```python
from build123d import *

# Parameters (mm, degrees)
SKETCH1_W           = 66.04
SKETCH1_H           = 147.574
BOSS_EXTRUDE1_DEPTH = 3.03784
SKETCH3_W           = 66.04
SKETCH3_H           = 3.03784
BOSS_EXTRUDE2_DEPTH = 16.51
SKETCH4_R           = 3.3782
CUT_EXTRUDE1_DEPTH  = 163.854183627
SKETCH5_R           = 2.5527
CUT_EXTRUDE2_DEPTH  = 3.03784
BASE_FLANGE1_START  = -66.04
BASE_FLANGE1_DEPTH  = 66.04
SKETCH11_R          = 3.3782
CUT_EXTRUDE3_DEPTH  = 163.854183627
SKETCH12_R          = 2.2479
CUT_EXTRUDE4_DEPTH  = 163.517528827
CUT_EXTRUDE6_DEPTH  = 1.51892
EDGE_FLANGE1_DEPTH  = 128.79832


# Read off the part's stored shape, not the designer's step: Base-Flange1
# Sheet-metal steps are written as plain solids
with BuildPart() as part:
    # Sketch1 → Boss-Extrude1 (new body)
    with BuildSketch(Plane.XY):
        with Locations((33.02, 73.787)):
            Rectangle(SKETCH1_W, SKETCH1_H)
    extrude(amount=BOSS_EXTRUDE1_DEPTH)

    # Sketch3 → Boss-Extrude2 (add)
    with BuildSketch(Plane.XY.offset(3.03784)):
        with Locations((33.02, 146.05508)):
            Rectangle(SKETCH3_W, SKETCH3_H)
        with Locations((33.02, 1.51892)):
            Rectangle(SKETCH3_W, SKETCH3_H)
    extrude(amount=BOSS_EXTRUDE2_DEPTH)

    # Sketch4 → Cut-Extrude1 (cut, through all)
    with BuildSketch(Plane.XZ):
        with Locations(Location((12.7, 12.68984, 0), (0, 0, 270))):
            Circle(SKETCH4_R)
        with Locations(Location((53.34, 12.68984, 0), (0, 0, 270))):
            Circle(SKETCH4_R)
    extrude(amount=-CUT_EXTRUDE1_DEPTH, mode=Mode.SUBTRACT)

    # Sketch5 → Cut-Extrude2 (cut)
    with BuildSketch(Plane.XY.offset(3.03784)):
        with Locations((46.99, 126.449057869)):
            Circle(SKETCH5_R)
        with Locations((19.05, 126.449057869)):
            Circle(SKETCH5_R)
        with Locations((6.35, 75.141057869)):
            Circle(SKETCH5_R)
        with Locations((59.69, 75.141057869)):
            Circle(SKETCH5_R)
    extrude(amount=-CUT_EXTRUDE2_DEPTH, mode=Mode.SUBTRACT)


with BuildPart() as body_2:
    # Base-Flange1 outline → Base-Flange1 (new body)
    with BuildSketch(Plane.ZY.offset(BASE_FLANGE1_START)):
        with BuildLine():
            ThreePointArc((1.51892, 4.94284), (2.52176295, 2.52176295), (4.94284, 1.51892))
            Line((4.94284, 1.51892), (19.54784, 1.51892))
            Line((19.54784, 1.51892), (19.54784, 3.03784))
            Line((19.54784, 3.03784), (4.94284, 3.03784))
            ThreePointArc((4.94284, 3.03784), (3.595801582, 3.595801582), (3.03784, 4.94284))
            Line((3.03784, 4.94284), (3.03784, 142.63116))
            ThreePointArc((3.03784, 142.63116), (3.595801582, 143.978198418), (4.94284, 144.53616))
            Line((4.94284, 144.53616), (19.54784, 144.53616))
            Line((19.54784, 144.53616), (19.54784, 146.05508))
            Line((19.54784, 146.05508), (4.94284, 146.05508))
            ThreePointArc((4.94284, 146.05508), (2.52176295, 145.05223705), (1.51892, 142.63116))
            Line((1.51892, 142.63116), (1.51892, 4.94284))
        make_face()
    extrude(amount=BASE_FLANGE1_DEPTH)

    # Sketch11 → Cut-Extrude3 (cut, through all)
    with BuildSketch(Plane.XZ):
        with Locations((53.34, 12.68984)):
            Circle(SKETCH11_R)
        with Locations((12.7, 12.68984)):
            Circle(SKETCH11_R)
    extrude(amount=-CUT_EXTRUDE3_DEPTH, mode=Mode.SUBTRACT)

    # Sketch12 → Cut-Extrude4 (cut, through all)
    with BuildSketch(Plane.XY.offset(3.03784)):
        with Locations((55.9637, 77.009977807)):
            Circle(SKETCH12_R)
        with Locations((9.8441, 77.009977807)):
            Circle(SKETCH12_R)
        with Locations((46.993900058, 128.317977807)):
            Circle(SKETCH12_R)
        with Locations((19.053900058, 128.317977807)):
            Circle(SKETCH12_R)
    extrude(amount=-CUT_EXTRUDE4_DEPTH, mode=Mode.SUBTRACT)

    # Sketch14 → Cut-Extrude6 (cut)
    with BuildSketch(Plane.XY.offset(3.03784)):
        with BuildLine():
            Line((21.301800058, 134.667977807), (21.301800058, 121.967977807))
            ThreePointArc((21.301800058, 121.967977807), (19.053900058, 119.720077807), (16.806000058, 121.967977807))
            Line((16.806000058, 121.967977807), (16.806000058, 134.667977807))
            ThreePointArc((16.806000058, 134.667977807), (19.053900058, 136.915877807), (21.301800058, 134.667977807))
        make_face()
        with BuildLine():
            Line((53.7158, 70.659977807), (53.7158, 83.359977807))
            ThreePointArc((53.7158, 83.359977807), (55.9637, 85.607877807), (58.2116, 83.359977807))
            Line((58.2116, 83.359977807), (58.2116, 70.659977807))
            ThreePointArc((58.2116, 70.659977807), (55.9637, 68.412077807), (53.7158, 70.659977807))
        make_face()
        with BuildLine():
            Line((49.241800058, 134.667977807), (49.241800058, 121.967977807))
            ThreePointArc((49.241800058, 121.967977807), (46.993900058, 119.720077807), (44.746000058, 121.967977807))
            Line((44.746000058, 121.967977807), (44.746000058, 134.667977807))
            ThreePointArc((44.746000058, 134.667977807), (46.993900058, 136.915877807), (49.241800058, 134.667977807))
        make_face()
        with BuildLine():
            Line((12.092, 83.359977807), (12.092, 70.659977807))
            ThreePointArc((12.092, 70.659977807), (9.8441, 68.412077807), (7.5962, 70.659977807))
            Line((7.5962, 70.659977807), (7.5962, 83.359977807))
            ThreePointArc((7.5962, 83.359977807), (9.8441, 85.607877807), (12.092, 83.359977807))
        make_face()
    extrude(amount=-CUT_EXTRUDE6_DEPTH, mode=Mode.SUBTRACT)

    # Edge-Flange1 section (across the edge) → Edge-Flange1 (add)
    with BuildSketch(Plane(origin=(67.945, 9.38784, 3.03784), x_dir=(-1, 0, 0), z_dir=(0, 1, 0))):
        with BuildLine():
            Line((-1.51892, 1.905), (-1.51892, 9.525))
            Line((-1.51892, 9.525), (0, 9.525))
            Line((0, 9.525), (0, 1.905))
            ThreePointArc((0, 1.905), (0.557961582, 0.557961582), (1.905, 0))
            Line((1.905, 0), (1.905, -1.51892))
            ThreePointArc((1.905, -1.51892), (-0.51607705, -0.51607705), (-1.51892, 1.905))
        make_face()
    edge_flange1 = extrude(amount=EDGE_FLANGE1_DEPTH)

    # Mirror1: Edge-Flange1 across plane
    add(edge_flange1.mirror(Plane(origin=(33.02, 0, 0), x_dir=(0, 0, 1), z_dir=(1, 0, 0))))


solid = body_2.part
```
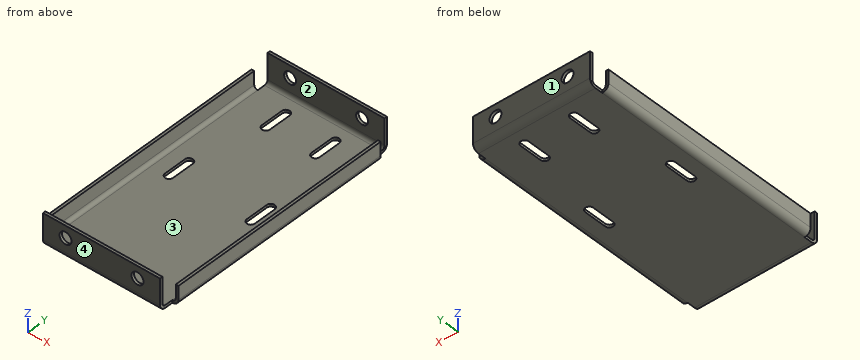
Input: part model. Units: mm. Frame: model coordinates. Face numbers are marked on the shaded views. A direction names the side the tool comes from. Give positions to 0.01 mm unless a question says otherwise; leave off trailing zeros. Order: outer loops, then holes, each group sorted by start corner. A loop starts at its lowest first (then second) coordinate and runs counter-clockwise, first axis right, second up. Notation, with made-up numbers: M -26.5,72.25 L 16.5,72.25 A28 cw 16.5,91.25 Z; hole C 41,68 d3. An arc over 180 degrees is marked long. Return JSON: item names as keys, results as strings.
Item 1: Cut plane B-B (x = 5). Return loops of the section in (y, z) (3 decimals).
Solutions:
{"outline": "M 1.519,4.943 A3.424 ccw 4.943,1.519 L 142.631,1.519 A3.424 ccw 146.055,4.943 L 146.055,19.548 L 144.536,19.548 L 144.536,4.943 A1.905 cw 142.631,3.038 L 4.943,3.038 A1.905 cw 3.038,4.943 L 3.038,19.548 L 1.519,19.548 Z"}
Item 2: Access query for the marked faces 1 and 2. Directions: +Z, -Z, +X, -X, +Y, -Y. A direction counts if a zero-diameter tool reaches every point of the face in a straight line with its end or side. Return the directions, or none.
Solutions:
{"face 1": "+Z, -Z, +X, -X, +Y", "face 2": "+Z, +X, -X"}
Item 3: Cut plane A-A (z = 14.25). Return loops of the section in (x, y), then the cut area to 3 significant figures.
Solutions:
{"outline": "M 0,1.52 L 9.7,1.52 L 9.7,3.04 L 0,3.04 Z; M 0,144.54 L 9.7,144.54 L 9.7,146.06 L 0,146.06 Z; M 15.7,1.52 L 50.34,1.52 L 50.34,3.04 L 15.7,3.04 Z; M 15.7,144.54 L 50.34,144.54 L 50.34,146.06 L 15.7,146.06 Z; M 56.34,1.52 L 66.04,1.52 L 66.04,3.04 L 56.34,3.04 Z; M 56.34,144.54 L 66.04,144.54 L 66.04,146.06 L 56.34,146.06 Z", "area": "164 mm^2"}
Item 4: Pull-direction query (X, two-part tool) for the marked faces 3 and 4; classes: +X half, -X half, draft (parallel to the pull), parting line (faces both ways), or undercut.
Solutions:
{"face 3": "undercut", "face 4": "draft"}
Item 5: Cut plane C-C (y = 51). Return loops of the section in (x, z) (3 decimals).
Solutions:
{"outline": "M -3.424,4.943 A3.424 ccw 0,1.519 L 66.04,1.519 A3.424 ccw 69.464,4.943 L 69.464,12.563 L 67.945,12.563 L 67.945,4.943 A1.905 cw 66.04,3.038 L 0,3.038 A1.905 cw -1.905,4.943 L -1.905,12.563 L -3.424,12.563 Z"}
Item 6: Ray query, probe 1 along Y at (x, z) = (20.5, 17.25); probe 2 along X at (y, z) = (127.5, 10.5) (3 decimals); probe 3 along Z at (x, y) = (41, 97.5). Return the intervals inside material, ascending.
Solutions:
{"probe 1": "1.52 to 3.04, 144.54 to 146.06", "probe 2": "-3.424 to -1.905, 67.945 to 69.464", "probe 3": "1.52 to 3.04"}
Item 7: First-contact query: P1, Ø8.5, axis at y = 142, z = 9.5, coming from the -X side; P2, Ø6, axis at x = 53.34, z = 12.69, coming from the -Y side; P3, Ø1.2, axis at y = 77.5, z = 2.5, coming from the +X side; P4, Ø8, axis at x = 46, y = 119.5, coming from the +Z side. Flat tips, straight axial feed; report the tip coordinate or a pass-through.
Solutions:
{"P1": "x = -3.42", "P2": "through", "P3": "x = 68.93", "P4": "z = 3.04"}
